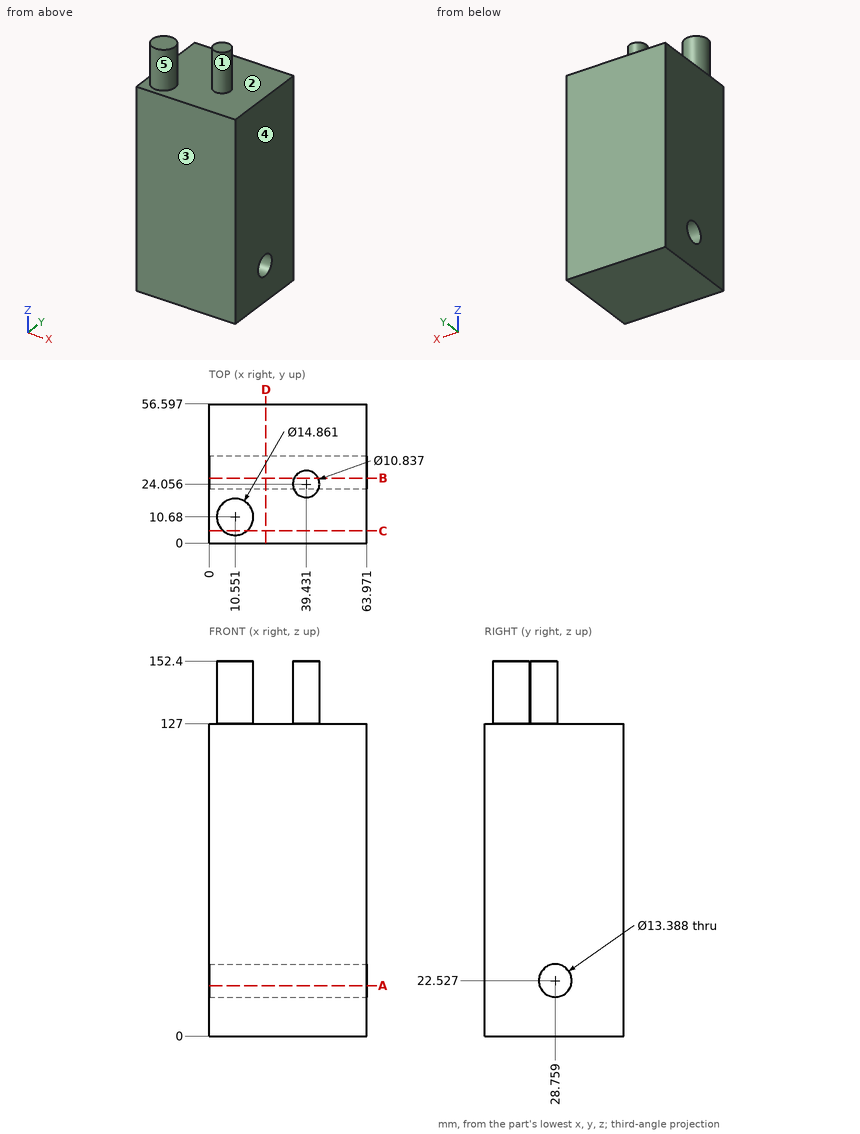
Job drawing, mm, ordinate dimensions from the low corner. One solid piece. A direction names the side the tool comes from. Coordinates: 2 decimals unless noted, no trailing zeros. Loops run counter-clockwise (first coordinate to the right, second up) from the corner with the lowest first, then second, coordinate; pieces in that order, holes last. Notation, with made-up numbers: (11.5, 29.25) -> (40.5, 29.25) arc R30 ccw to (40.5, 67.25) -> close; hole circle Ø6 at (80, 60). An arc over 180 degrees is marked (long way). One line per item, written item: value.
1. Slice it at A-A on z = 20.5. Write the cut outline in (x, y), and give its area (3 significant figures).
Answers:
outline: (0, 0) -> (63.97, 0) -> (63.97, 22.38) -> (0, 22.38) -> close; (0, 35.14) -> (63.97, 35.14) -> (63.97, 56.6) -> (0, 56.6) -> close
area: 2,800 mm^2
2. Pull direction Y, two halves, no side cores. Call the marked faces 1, 2 and 3: pulls with the +Y half, pulls with the -Y half, needs draft (parallel to the pull), parting line crosses it, or undercut.
Answers:
face 1: parting line crosses it
face 2: needs draft
face 3: pulls with the -Y half
3. Slice it at D-D on x = 23. Write the cut outline in (y, z), and give its area (3 significant figures).
Answers:
outline: (0, 0) -> (56.6, 0) -> (56.6, 127) -> (0, 127) -> close; hole circle Ø13.39 at (28.76, 22.53)
area: 7,050 mm^2
4. Slice it at B-B on y = 26.5. Write the cut outline in (x, z) (1 decimal), and give its area (3 significant figures).
Answers:
outline: (0, 0) -> (64, 0) -> (64, 16.2) -> (0, 16.2) -> close; (0, 28.8) -> (64, 28.8) -> (64, 127) -> (44.3, 127) -> (44.3, 152.4) -> (34.6, 152.4) -> (34.6, 127) -> (0, 127) -> close
area: 7,560 mm^2
5. Drill centre lines: line 1 (Z direction, x = 43, y = 46.5); line 2 (Y direction, x = 59, z = 17) (1 decimal); line 3 (Y direction, x = 40, z = 21). Where is each one in solid material? Low to high. Write a range as [from, to].
Answers:
line 1: z = [0, 127]
line 2: y = [0, 25], [32.5, 56.6]
line 3: y = [0, 22.24], [35.28, 56.6]
6. Which spindle directions (+Z, -Z, +X, -X, +Y, -Y) get a long thin tool onto all of the face, cutting with end or side? Do the marked faces 4 and 5. Say none if no direction does.
Answers:
face 4: +Z, -Z, +X, +Y, -Y
face 5: +Z
7. Slice it at C-C on y = 5. Write the cut outline in (x, z).
Answers:
outline: (0, 0) -> (63.97, 0) -> (63.97, 127) -> (15.34, 127) -> (15.34, 152.4) -> (5.76, 152.4) -> (5.76, 127) -> (0, 127) -> close
